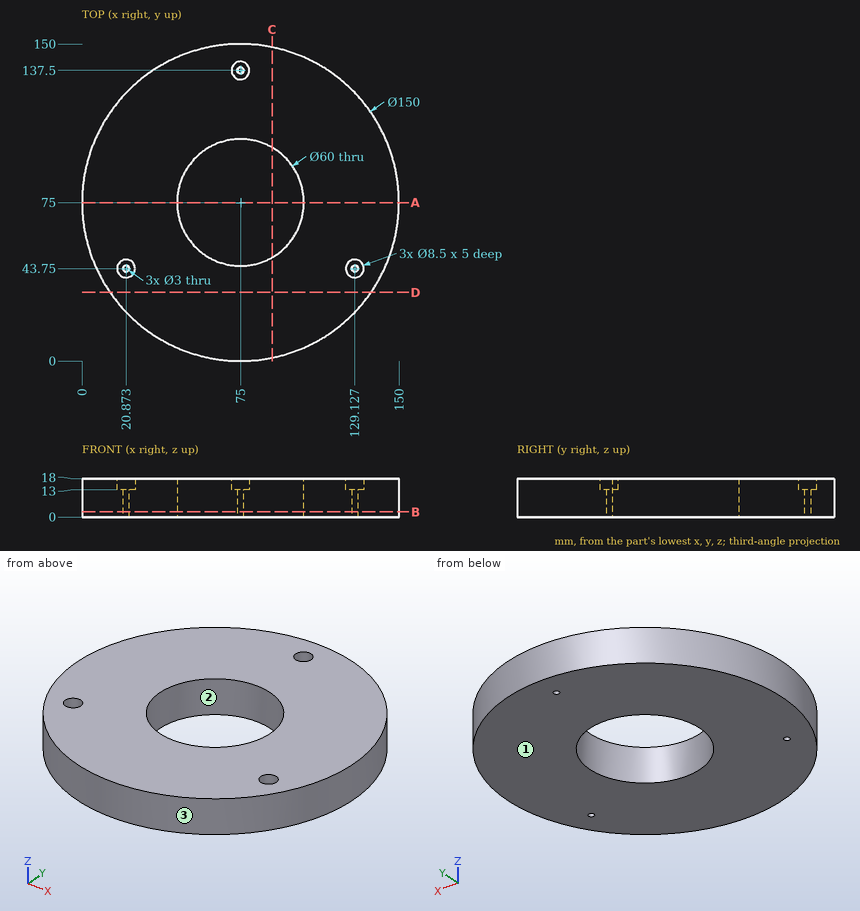
Design review of the part shown in the three views and the two pictorial views. Dimensions are in mm from the part's minimum x, y and z. Give positions to 0.01 mm unless a question says otherwise; leave off trailing zeros. Loops run counter-clockwise (first coordinate to the right, second up) from the corner with the lowest first, then second, coordinate; pieces in that order, holes last. Notation, with made-up numbers: (28, -21) -> (74, -21) arc R22 ccw to (74, 13) -> close; hole circle Ø2 at (4, -7.5). An arc over 180 degrees is marked (long way). Answer as a JSON object with one key per item and string values. Group by question number.
Q1. Wall thickness on line 1 along X through (y, z) = (43.75, 9.25) (1 decimal); line 2 along Y through (x, z) = (75, 10.25); line 3 along Y through (x, z) = (75, 14.15): over which ranges is each line inside the solid? List them lowest first.
Q2. Take a section at B-B (z = 2.5). Write out the cut boundary in (x, y).
Q3. Insertion check: pin 1 (9.5 mm diameter, centred on x = 127, y = 42.5, fed in from +Z); pin 2 (6 mm diameter, centred on x = 68.5, z = 11.5, fed in from -Y); pin 3 (3 mm diameter, centred on x = 116, z = 3.5, fed in from -Y) (1 decimal); pin 4 (5 mm diameter, centred on x = 75, y = 137.5, fed in from +Z). Each pin has a flat end and moves straight along its axis. Give the tip position at first contact, or say it passes through.
Q4. Take a section at C-C (x = 90). Write out the cut boundary in (y, z) (1 decimal).
Q5. Take a section at D-D (y = 32.5). Write out the cut boundary in (x, z), plus the area to 3 significant figures.
Q6. Take a section at A-A (y = 75). Write out the cut boundary in (x, z).
Q7. Draft analysis for pull direction X (two halves, no side actions). For the marked faces 1, 2 and 3, state which applies: pulls with the +X half, pulls with the -X half, needs draft (parallel to the pull), parting line crosses it, or undercut.
Answer below:
{
 "1": {"line 1": "x = 6.8 to 19.4, 22.4 to 127.6, 130.6 to 143.2", "line 2": "y = 0 to 45, 105 to 136, 139 to 150", "line 3": "y = 0 to 45, 105 to 133.25, 141.75 to 150"},
 "2": {"outline": "circle Ø150 at (75, 75); hole circle Ø3 at (20.87, 43.75); hole circle Ø60 at (75, 75); hole circle Ø3 at (75, 137.5); hole circle Ø3 at (129.13, 43.75)"},
 "3": {"pin 1": "stops at z = 18", "pin 2": "stops at y = 0.08", "pin 3": "stops at y = 11.2", "pin 4": "stops at z = 13"},
 "4": {"outline": "(1.5, 0) -> (49, 0) -> (49, 18) -> (1.5, 18) -> close; (101, 0) -> (148.5, 0) -> (148.5, 18) -> (101, 18) -> close"},
 "5": {"outline": "(13.2, 0) -> (136.8, 0) -> (136.8, 18) -> (13.2, 18) -> close", "area": "2,220 mm2"},
 "6": {"outline": "(0, 0) -> (45, 0) -> (45, 18) -> (0, 18) -> close; (105, 0) -> (150, 0) -> (150, 18) -> (105, 18) -> close"},
 "7": {"face 1": "needs draft", "face 2": "undercut", "face 3": "parting line crosses it"}
}
